Check sheet for the modelled part. Datum: model origin and axes. Units: mm. A direction names the side the tool comes from. Round coordinates to 2 decimals unless told otherwise and drop trailing zeros. Order: outer loops, then holes, each group sorted by start corner. A loop starts at its lowest first (then second) coordinate and runs counter-clockwise, first axis right, second up.
Q1. Depth check by flat-ended pin: P1, Ø6, axis at x = 5.5, y = -14, coming from the +Z side; P2, Ø6.5, axis at x = 11, y = -18, coming from the +Z side; P3, Ø6.5, axis at y = -7.5, z = 16, coming from the +X side; P4, Ø2, axis at x = 12.5, y = -14, coming from the -Z side (3 decimals). Enter the tip coordinate at first touch or a pass-through.
Q2. Cross-section at B-B on x = 12.5. Record the cut outline in (y, z), then the cut area to 3 significant figures.
Q3. Cross-section at D-D on z = 8.5. Record the cut outline in (x, y), then the cut area to 3 significant figures.
Q4. Cross-section at A-A on z = 12.5. Record the cut outline in (x, y).
Q5. Mould release check, pull along Y, two halves, no side actions. Record for faces 1 (the cylindrical face through (2.871, -12.476, 11.868)), 2 (the flat face through (2, -14, 25)), 3 (the flat face through (3, 0, 8)): +Y half, -Y half, draft (parallel to the pull), parting line (faces both ways), or undercut.
Q6. Set-up check for faces 4 (the flat face through (10, -11, 0)), 5 (the flat face through (15, -14, 4)): record each of +Z, -Z, +X, -X, +Y, -Y from which the full face is reachable in a straight line by a thin tool's end or side.
Q7. Cross-section at C-C on y = -18.75. Record the cut outline in (x, z), then the cut area to 3 significant figures.
Q8. Scan lines: probe 1 along X at (y, z) = (-14, 2.8); probe 2 along Y at (x, z) = (3.2, 12.5). Record each from-to range of solid material in increasing order.
from build123d import *

# Parameters (mm, degrees)
F1_DEPTH       = 28
F3_D           = 3.3
F3_DEPTH       = 40
F3_CSINK_D     = 6.72
F3_CSINK_ANGLE = 90
F3_TIP         = 0.9914200214
F5_D           = 3.3
F5_DEPTH       = 40
F5_CSINK_D     = 6.72
F5_CSINK_ANGLE = 90
F5_TIP         = 0.9914200214


with BuildPart() as f1:
    # F0 (on Front) → F1 (new body)
    with BuildSketch(Plane.XZ):
        Polygon((0, 4), (0, 0), (4, 0), (25, 0), (25, 4), (4, 4), (4, 25), (0, 25), align=None)
    extrude(amount=F1_DEPTH)

    # F3
    with Locations(Plane(origin=(0, 0, 0), x_dir=(0, -1, 0), z_dir=(-1, 0, 0))):
        with Locations((14, 12.5)):
            CounterSinkHole(F3_D / 2, F3_CSINK_D / 2, depth=F3_DEPTH, counter_sink_angle=F3_CSINK_ANGLE)
            with Locations((0, 0, -(F3_DEPTH + F3_TIP / 2))):  # 118° drill point
                Cone(0, F3_D / 2, F3_TIP, mode=Mode.SUBTRACT)

    # F5
    with Locations(Plane(origin=(0, 0, 0), x_dir=(1, 0, 0), z_dir=(0, 0, -1))):
        with Locations((12.5, 14)):
            CounterSinkHole(F5_D / 2, F5_CSINK_D / 2, depth=F5_DEPTH, counter_sink_angle=F5_CSINK_ANGLE)
            with Locations((0, 0, -(F5_DEPTH + F5_TIP / 2))):  # 118° drill point
                Cone(0, F5_D / 2, F5_TIP, mode=Mode.SUBTRACT)


solid = f1.part
Results found:
1. P1: stops at z = 25
1. P2: stops at z = 4
1. P3: stops at x = 4
1. P4: passes through
2. outline: (-28, 0) - (-17.36, 0) - (-15.65, 1.71) - (-15.65, 4) - (-28, 4) - close; (-12.35, 1.71) - (-10.64, 0) - (0, 0) - (0, 4) - (-12.35, 4) - close
2. area: 95.9 mm2
3. outline: (0, -28) - (4, -28) - (4, 0) - (0, 0) - close
3. area: 112 mm2
4. outline: (0, -28) - (4, -28) - (4, -15.65) - (1.71, -15.65) - (0, -17.36) - close; (0, -10.64) - (1.71, -12.35) - (4, -12.35) - (4, 0) - (0, 0) - close
5. face 1: undercut
5. face 2: draft
5. face 3: +Y half
6. face 4: -Z, +X, -X, +Y, -Y
6. face 5: +Z, +X, +Y, -Y
7. outline: (0, 0) - (25, 0) - (25, 4) - (4, 4) - (4, 25) - (0, 25) - close
7. area: 184 mm2
8. probe 1: x = 0 to 10.85, 14.15 to 25
8. probe 2: y = -28 to -15.65, -12.35 to 0
